Read the model definition and answer for the solid it produces. Units are mm, in the model's axes. A direction names the side the tool comes from. Coordinates: 2 decimals unless noted, no trailing zeros. Order: outer loops, then holes, each group sorted by start corner. A loop starts at its lowest first (then second) coordinate and runs counter-clockwise, first axis right, second up.
Autodesk Inventor part; units mm, degrees
ref_plane "YZ Plane" through (0, 0, 0) normal (1, 0, 0) x (0, 1, 0)
ref_plane "XZ Plane" through (0, 0, 0) normal (0, 1, 0) x (-1, 0, 0)
ref_plane "XY Plane" through (0, 0, 0) normal (0, 0, 1) x (1, 0, 0)
sketch "Skizze1" plane through (0, 0, 0) normal (0, 0, 1) x (1, 0, 0)
  circle A0 centre (0, 0) radius 25 construction
  circle A1 centre (0, 0) radius 30 construction
  line L0 (-24.955, 1.5) -> (-44.2874, 1.5)
  line L1 (-44.2874, 1.5) -> (-44.2874, 6.5)
  line L2 (-44.2874, 6.5) -> (-29.2874, 6.5)
  line L3 (-24.955, -1.5) -> (-44.2874, -1.5)
  line L4 (-44.2874, -1.5) -> (-44.2874, -6.5)
  line L5 (-44.2874, -6.5) -> (-29.2874, -6.5)
  arc A2 (-29.2874, -6.5) -> (-29.2874, 6.5) centre (0, 0) ccw
  arc A3 (-24.955, -1.5) -> (-24.955, 1.5) centre (0, 0) ccw
  line L6 (-59.1448, 0) -> (44.8575, 0) construction
  dimension "d0" = 50
  dimension "d1" = 60
  dimension "d2" = 5
  dimension "d4" = 3
  dimension "d5" = 15
extrude "Extrusion1" add sketch "Skizze1" along normal mid plane 20
sketch "Skizze2" plane through (-44.2874, 6.5, 10) normal (0, 1, 0) x (1, 0, 0)
  line L0 (0, 20) -> (15, 0) construction
  line L1 (15, 20) -> (0, 0) construction
  line L2 (2.5, 12.8868) -> (7.5, 15.7735)
  line L3 (7.5, 15.7735) -> (12.5, 12.8868)
  line L4 (12.5, 12.8868) -> (12.5, 7.1132)
  line L5 (12.5, 7.1132) -> (7.5, 4.2265)
  line L6 (7.5, 4.2265) -> (2.5, 7.1132)
  line L7 (2.5, 7.1132) -> (2.5, 12.8868)
  circle A0 centre (7.5, 10) radius 3.25
  point P0 (44.2874, 10)
  dimension "d8" = 10
  dimension "d9" = 6.5
extrude "Extrusion2" cut sketch "Skizze2" against normal through all contours A0
extrude "Extrusion3" cut sketch "Skizze2" against normal blind 3
properties part number "Zyklon_Schelle"
Q1. Each of these flat-tipped pins is pushed along its axis until it touches: P1, Ø11, axis at x = -35, z = 2.5, coming from the +Y side; P2, Ø2, axis at y = -11.5, z = 5.5, coming from the +X side; P3, Ø1, axis at x = -14, y = -19.5, coming from the +Z side; P4, Ø5, axis at x = -22.5, z = 2, coming from the -Y side. Where does it stop, or does it pass through?
Q2. Which of the six approach directions +Z, -Z, +X, -X, +Y, -Y give full straight-line access (tool end or side, diameter ignored) to faces 1 (the flat face through (-24, 9, 10)), 2 (the flat face through (-40.2, -6.5, -0.1)), 3 (the flat face through (-32, 1.5, 0)), 4 (the cylindrical face through (-40.034, -3.965, -0.143)), 5 (the flat face through (-39.32, 5.02, -4.31))?
Q3. The part is cut by section A-A, the plane x = 0. Determine the outline of the cut face in (y, z).
Q4. Determine the mould class of faces 6 (the flat face through (-32, -1.5, 0)), 7 (the flat face through (-42, 6.5, 0)), 8 (the flat face through (-44.287, -4, 0)) for opening direction Y: +Y half, -Y half, draft (parallel to the pull), parting line (faces both ways), or undercut.
Q5. The part is cut by section B-B, the plane y = 13. Determine the outline of the cut face in (x, z).
Q6. The part is cut by section D-D, the plane y = 0. Determine the outline of the cut face in (x, z), then the cut area to 4 significant figures.
Q7. Straight lines are drawn through the part: L1, parallel to Y at x = 0, z = 0; L2, parallel to X at y = 3.05, z = 0; L3, parallel to X at y = -4.45, z = 0. For each, find the intervals that lie inside material, in ascending order.
Q8. The part is cut by section C-C, the plane z = 1.75. Determine the outline of the cut face in (x, y) (3 decimals), then the cut area to 4 significant figures.
Computed values:
1. P1: stops at y = 6.5
1. P2: stops at x = 28.1
1. P3: passes through
1. P4: stops at y = -22.36
2. face 1: +Z, +X, -X, +Y, -Y
2. face 2: +Z, -Z, -X, -Y
2. face 3: +Z, -Z, -X
2. face 4: +Y, -Y
2. face 5: +Y
3. outline: (-30, -10) - (-25, -10) - (-25, 10) - (-30, 10) - close; (25, -10) - (30, -10) - (30, 10) - (25, 10) - close
4. face 6: undercut
4. face 7: +Y half
4. face 8: draft
5. outline: (-27.04, -10) - (-21.35, -10) - (-21.35, 10) - (-27.04, 10) - close; (21.35, -10) - (27.04, -10) - (27.04, 10) - (21.35, 10) - close
6. outline: (25, -10) - (30, -10) - (30, 10) - (25, 10) - close
6. area: 100.0 mm2
7. L1: y = -30 to -25, 25 to 30
7. L2: x = -44.29 to -40.04, -33.54 to -24.81, 24.81 to 29.84
7. L3: x = -44.29 to -40.04, -33.54 to -24.6, 24.6 to 29.67
8. outline: (-44.287, -6.5) - (-39.526, -6.5) - (-39.526, -1.5) - (-44.287, -1.5) - close; (-44.287, 1.5) - (-39.526, 1.5) - (-39.526, 3.5) - (-41.787, 3.5) - (-41.787, 6.5) - (-44.287, 6.5) - close; (-34.049, -6.5) - (-29.287, -6.5) arc R30 ccw (long way) to (-29.287, 6.5) - (-31.787, 6.5) - (-31.787, 3.5) - (-34.049, 3.5) - (-34.049, 1.5) - (-24.955, 1.5) arc R25 cw (long way) to (-24.955, -1.5) - (-34.049, -1.5) - close
8. area: 926.5 mm2
